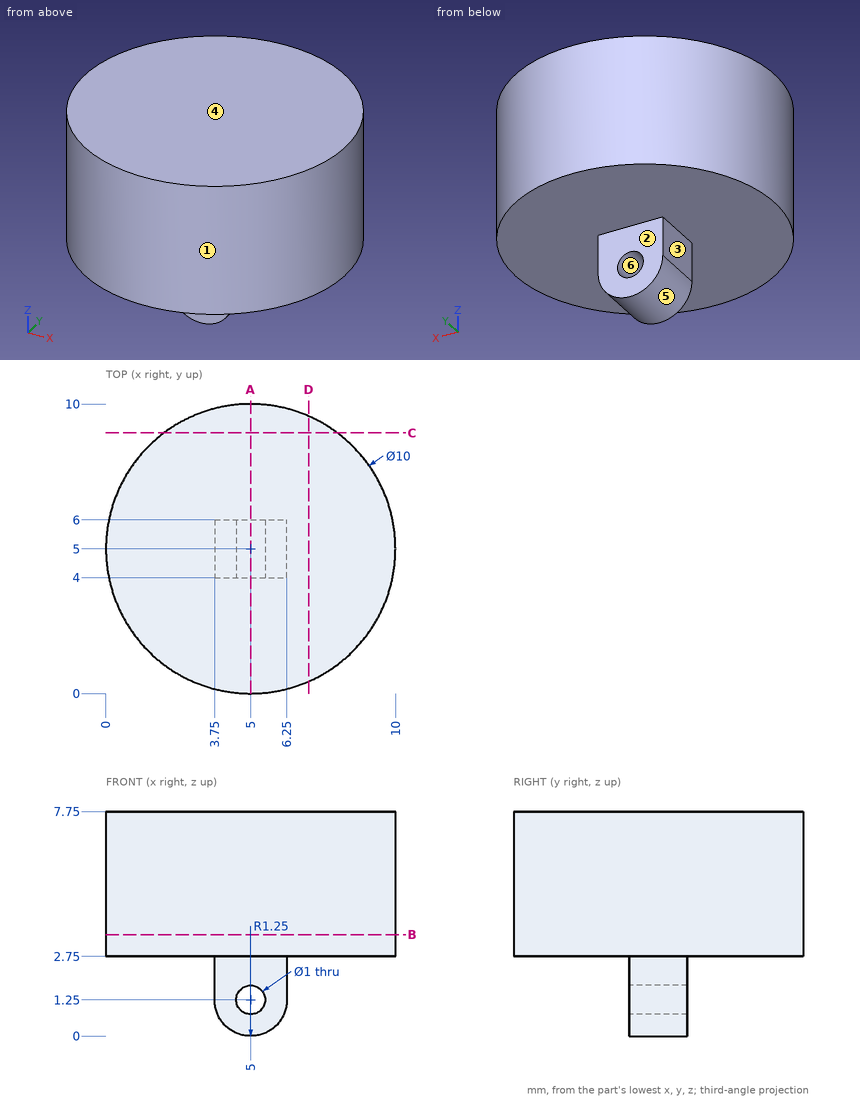
For this review, use the dimensioned drawing (mm, ordinates from the lowest corner) and the shaded views. A direction names the side the tool comes from. Give positions to 0.01 mm unless a question says otherwise; leave off trailing zeros. Order: outer loops, then holes, each group sorted by start corner. A loop starts at its lowest first (then second) coordinate and runs counter-clockwise, first axis right, second up. Notation, with made-up numbers: (53.5, -38.75) - (107.5, -38.75) arc R19 ccw to (107.5, -33.75) - close; hole circle Ø5 at (83, 67.25). An arc over 180 degrees is marked (long way). Use CSV: the item, a comma, the result in double quotes. Start each with the question number.
Q1. We need section B-B, the plane z = 3.5. Write out the cut boundary in (x, y).
Q2. Tool access review of the marked faces 1 and 2: name each direction out of +Z, -Z, +X, -X, +Y, -Y from which nothing blocks a thin tool from reaching the whole face with its end or side.
Q3. We need section D-D, the plane x = 7. Write out the cut boundary in (y, z).
Q4. We need section C-C, the plane y = 9. Write out the cut boundary in (x, z), and give its area (3 significant figures).
Q5. We need section A-A, the plane x = 5. Write out the cut boundary in (y, z).
Q6. The part is to be moulded in two halves that separate along Z. For the marked faces 3, 4, 5 and 6, say which applies: +Z half, -Z half, draft (parallel to the pull), parting line (faces both ways), or undercut.
Q7. Clearance check with flat-ended pins moving along their axes: pin 1 Ø1 at (x, z) = (1.5, 4.5) entering from +Y; pin 2 Ø1.2 at (x, z) = (5.5, 2) entering from +Y. State where each tip first meets the part, or that it passes through.
Q8. To check wall thickness, follow line 1 along X through (y, z) = (4.5, 1.25); line 2 along Z through (x, y) = (1.5, 4.75); line 3 along X through (y, z) = (6.75, 3.25). State the ranges of each line that lie inside material, in increasing order. Write a range as [from, to].
Outcome:
1,outline,"circle Ø10 at (5, 5)"
2,face 1,"+Z, -Z"
2,face 2,"-Z, +X, -X, +Y"
3,outline,"(0.42, 2.75) - (9.58, 2.75) - (9.58, 7.75) - (0.42, 7.75) - close"
4,outline,"(2, 2.75) - (8, 2.75) - (8, 7.75) - (2, 7.75) - close"
4,area,"30.0 mm^2"
5,outline,"(0, 2.75) - (4, 2.75) - (4, 1.75) - (6, 1.75) - (6, 2.75) - (10, 2.75) - (10, 7.75) - (0, 7.75) - close; (4, 0) - (6, 0) - (6, 0.75) - (4, 0.75) - close"
6,face 3,"draft"
6,face 4,"+Z half"
6,face 5,"-Z half"
6,face 6,"undercut"
7,pin 1,"stops at y = 9"
7,pin 2,"stops at y = 6"
8,line 1,"x = [3.75, 4.5], [5.5, 6.25]"
8,line 2,"z = [2.75, 7.75]"
8,line 3,"x = [0.32, 9.68]"
